```python
from build123d import *

# Parameters (mm, degrees)
SKETCH1_R           = 48
SKETCH1_R_2         = 10
BOSS_EXTRUDE1_DEPTH = 10
CUT_EXTRUDE1_START  = -1.5
SKETCH2_R           = 11
CUT_EXTRUDE1_DEPTH  = 7.5
SKETCH3_R           = 43
SKETCH3_R_2         = 15
CUT_EXTRUDE2_DEPTH  = 8
SKETCH4_R           = 13.5
CUT_EXTRUDE3_DEPTH  = 8
FILLET1_START       = 2
FILLET1_OUTLINE_R   = 43
FILLET1_OUTLINE_R_2 = 13.5
FILLET1_OUTLINE_R_3 = 15
FILLET1_DEPTH       = 8.0000001


with BuildPart() as part:
    # Sketch1 → Boss-Extrude1 (new body)
    with BuildSketch(Plane.XY):
        Circle(SKETCH1_R)
        Circle(SKETCH1_R_2, mode=Mode.SUBTRACT)
    extrude(amount=BOSS_EXTRUDE1_DEPTH)

    # Sketch2 → Cut-Extrude1 (cut)
    with BuildSketch(Plane.XY.offset(10).offset(CUT_EXTRUDE1_START)):
        Circle(SKETCH2_R)
    extrude(amount=-CUT_EXTRUDE1_DEPTH, mode=Mode.SUBTRACT)

    # Sketch3 → Cut-Extrude2 (cut)
    with BuildSketch(Plane.XY.offset(10)):
        Circle(SKETCH3_R)
        Circle(SKETCH3_R_2, mode=Mode.SUBTRACT)
    extrude(amount=-CUT_EXTRUDE2_DEPTH, mode=Mode.SUBTRACT)

    # Sketch4 → Cut-Extrude3 (cut)
    with BuildSketch(Plane.XY.offset(2)):
        with Locations((-21.923747427, -19.362639251)):
            Circle(SKETCH4_R)
        with Locations((-25.189774768, 14.867338267)):
            Circle(SKETCH4_R)
        with Locations((6.355610451, 28.551159623)):
            Circle(SKETCH4_R)
        with Locations((29.117758046, 2.778248798)):
            Circle(SKETCH4_R)
        with Locations((11.640153697, -26.834107436)):
            Circle(SKETCH4_R)
    extrude(amount=-CUT_EXTRUDE3_DEPTH, mode=Mode.SUBTRACT)

    # Fillet1: read off the stored shape, not the designer's step
    # Fillet1 outline → Fillet1 (add)
    with BuildSketch(Plane.XY.offset(FILLET1_START)):
        Circle(FILLET1_OUTLINE_R)
        with Locations((-21.923747427, -19.362639251)):
            Circle(FILLET1_OUTLINE_R_2, mode=Mode.SUBTRACT)
        with Locations((11.640153697, -26.834107436)):
            Circle(FILLET1_OUTLINE_R_2, mode=Mode.SUBTRACT)
        with Locations((-25.189774768, 14.867338267)):
            Circle(FILLET1_OUTLINE_R_2, mode=Mode.SUBTRACT)
        Circle(FILLET1_OUTLINE_R_3, mode=Mode.SUBTRACT)
        with Locations((29.117758046, 2.778248798)):
            Circle(FILLET1_OUTLINE_R_2, mode=Mode.SUBTRACT)
        with Locations((6.355610451, 28.551159623)):
            Circle(FILLET1_OUTLINE_R_2, mode=Mode.SUBTRACT)
    extrude(amount=FILLET1_DEPTH)

    # Fillet1 2 outline → Fillet1 2 (revolve, cut)
    with BuildSketch(Plane.XZ):
        with BuildLine():
            ThreePointArc((15, 10), (18.473403651, 4.254033308), (24.797958971, 2))
            Line((24.797958971, 2), (33.202041029, 2))
            ThreePointArc((33.202041029, 2), (39.526596349, 4.254033308), (43, 10))
            Line((43, 10), (15, 10))
        make_face()
    revolve(axis=Axis((0, 0, 0), (0, 0, 1)), mode=Mode.SUBTRACT)


solid = part.part
```
Here's how the part is built. I have some questions about the finished solid (model axes, mm). A direction names the side the tool comes from. Round coordinates to 2 decimals unless told otherwise and drop trailing zeros. Loops run counter-clockwise (first coordinate to the right, second up) from the corner with the lowest first, then second, coordinate; pieces in that order, holes last. Notation, with made-up numbers: (-19.5, 55.25) -> (18.5, 55.25) arc R11 ccw to (18.5, 62.25) -> close; hole circle Ø7 at (77, -13). An arc over 180 degrees is marked (long way). Answer as CSV lines item,"result".
1. For pin 1 (2 mm diameter, centred on y = -37, z = 8, fed in from -X); pin 2 (21.5 mm diameter, centred on x = 29.12, y = 2.78, fed in from -Z); pin 3 (5 mm diameter, centred on y = 23, z = 3.5, fed in from +X); pin 4 (5 mm diameter, centred on x = -3.5, z = 5, fed in from +Y), each with a flat end and sliding along its axis, tell me the tip position at first contact or that it passes through.
Final values:
pin 1,"stops at x = -31.75"
pin 2,"passes through"
pin 3,"stops at x = 43.4"
pin 4,"stops at y = 47.99"
2. Thinking about a two-plate mould opening in Y: for faces 4 (the face through (-2.38, -10.74, 4.8)), 5 (the face through (-39.3, 18, 10)), 6 (the face through (2, -10, 8.5)), 7 (the face through (-47.954, 2.11, 4.93)), which applies, released by +Y, released by -Y, zero draft, split by the parting line, or undercut?
Final values:
face 4,"undercut"
face 5,"zero draft"
face 6,"undercut"
face 7,"split by the parting line"
3. If we section it at B-B on y = 0: Please give me the cut outline in (x, z).
Final values:
outline,"(-48, 0) -> (-10, 0) -> (-10, 1) -> (-11, 1) -> (-11, 8.5) -> (-10, 8.5) -> (-10, 10) -> (-15, 10) arc R10 cw to (-24.8, 2) -> (-33.2, 2) arc R10 cw to (-43, 10) -> (-48, 10) -> close; (10, 0) -> (15.91, 0) -> (15.91, 7.42) arc R10 cw to (15, 10) -> (10, 10) -> (10, 8.5) -> (11, 8.5) -> (11, 1) -> (10, 1) -> close; (42.33, 0) -> (48, 0) -> (48, 10) -> (43, 10) arc R10 cw to (42.33, 7.91) -> close"
4. Which directions (+Z, -Z, +X, -X, +Y, -Y) give clear straight access to the entire face, cutting with the end or side of a thin tool? Please do faces 1 (the face through (2, -10, 1)), 2 (the face through (23, 19, 2)), 3 (the face through (-1, 11, 0)).
Final values:
face 1,"none"
face 2,"+Z"
face 3,"-Z, +X, -X, +Y, -Y"
5. If we section it at C-C on x = -18: Count the separate pieces of the cut face and the enclosed holes in it, plus the area to 3 significant figures.
Final values:
separate pieces,"3"
enclosed holes,"0"
area,"235 mm^2"
6. If I drill on L1, parallel to X at y = 1, z = 0.75; L2, parallel to Y at x = -7.5, z = 7.75; L3, parallel to Y at x = 0, z = 0.5, over which ranges is the centre line in solid material (lowest first)?
Final values:
L1,"x = -47.99 to -9.95, 9.95 to 15.74, 42.5 to 47.99"
L2,"y = -47.41 to -41.58, -13.85 to -8.05, 8.05 to 13.85, 41.58 to 47.41"
L3,"y = -48 to -33.67, -20 to -10, 10 to 16.64, 40.46 to 48"
7. If we section it at A-A on z = 5.25: Please give me the cut outline in (x, y), plus the area to 3 significant figures.
Final values:
outline,"circle Ø96 at (0, 0); (-16.9, 4.21) arc R17.42 ccw to (-15.8, -7.33) arc R13.5 cw to (-9.23, -14.78) arc R17.42 ccw to (2.09, -17.29) arc R13.5 cw to (11.2, -13.34) arc R17.42 ccw to (17.09, -3.36) arc R13.5 cw to (16.15, 6.53) arc R17.42 ccw to (8.48, 15.22) arc R13.5 cw to (-1.22, 17.38) arc R17.42 ccw to (-11.85, 12.76) arc R13.5 cw to start; hole (-38.52, 12.76) arc R40.58 ccw to (-35.42, -19.81) arc R13.5 ccw to (-24.04, -32.7) arc R40.58 ccw to (7.9, -39.8) arc R13.5 ccw to (23.67, -32.96) arc R40.58 ccw to (40.3, -4.79) arc R13.5 ccw to (38.66, 12.32) arc R40.58 ccw to (17.01, 36.84) arc R13.5 ccw to (0.23, 40.58) arc R40.58 ccw to (-29.78, 27.56) arc R13.5 ccw to start; hole circle Ø22 at (0, 0)"
area,"2,450 mm^2"
